```python
from build123d import *

# Parameters (mm, degrees)
BOSS_EXTRUDE1_DEPTH     = 5
BOSS_EXTRUDE2_DEPTH     = 2.5
CUT_EXTRUDE1_DEPTH      = 150.653904127
CUT_EXTRUDE1_DEPTH_BACK = 150.653904127


with BuildPart() as part:
    # Sketch1 → Boss-Extrude1 (new, symmetric)
    # profile 1 of 2: a face of its own
    with BuildSketch(Plane.XY):
        with BuildLine():
            Line((56.958357345, 16.35690948), (91.94062397, 26.262392372))
            ThreePointArc((91.94062397, 26.262392372), (58.546836742, 40.020208922), (27.617225647, 21.371302811))
            ThreePointArc((27.617225647, 21.371302811), (21.454195768, 0), (27.617225647, -21.371302811))
            ThreePointArc((27.617225647, -21.371302811), (58.546836742, -40.020208922), (91.94062397, -26.262392372))
            Line((91.94062397, -26.262392372), (107.630769277, -4.631577729))
            Line((107.630769277, -4.631577729), (66.221512803, -16.35690948))
            ThreePointArc((66.221512803, -16.35690948), (45.233025594, -4.631577729), (56.958357345, 16.35690948))
        make_face()
    # profile 2 of 2: a face of its own
    with BuildSketch(Plane.XY):
        with BuildLine():
            ThreePointArc((27.617225647, -21.371302811), (21.454195768, 0), (27.617225647, 21.371302811))
            ThreePointArc((27.617225647, 21.371302811), (20.358110781, 14.513813118), (10.688318885, 12.02081528))
            Line((10.688318885, 12.02081528), (-112.81430605, 12.02081528))
            ThreePointArc((-112.81430605, 12.02081528), (-114.76520927, 12.212962476), (-116.641140374, 12.782019955))
            Line((-116.641140374, 12.782019955), (-126.824245004, 17))
            Line((-126.824245004, 17), (-138.845060284, 12.02081528))
            Line((-138.845060284, 12.02081528), (-143.824245004, 0))
            Line((-143.824245004, 0), (-138.845060284, -12.02081528))
            Line((-138.845060284, -12.02081528), (-126.824245004, -17))
            Line((-126.824245004, -17), (-116.641140374, -12.782019955))
            ThreePointArc((-116.641140374, -12.782019955), (-114.76520927, -12.212962476), (-112.81430605, -12.02081528))
            Line((-112.81430605, -12.02081528), (10.688318885, -12.02081528))
            ThreePointArc((10.688318885, -12.02081528), (20.358110781, -14.513813118), (27.617225647, -21.371302811))
        make_face()
        with BuildLine():
            ThreePointArc((-61.622122108, -6.728166576), (-68.350288684, 0), (-61.622122108, 6.728166576))
            Line((-61.622122108, 6.728166576), (-32.694798011, 6.728166576))
            ThreePointArc((-32.694798011, 6.728166576), (-25.966631435, 0), (-32.694798011, -6.728166576))
            Line((-32.694798011, -6.728166576), (-61.622122108, -6.728166576))
        make_face(mode=Mode.SUBTRACT)
    extrude(amount=BOSS_EXTRUDE1_DEPTH, both=True)

    # Sketch1_3 → Boss-Extrude2 (add, symmetric)
    with BuildSketch(Plane.XY):
        with BuildLine():
            Line((-61.622122108, -6.728166576), (-32.694798011, -6.728166576))
            ThreePointArc((-32.694798011, -6.728166576), (-25.966631435, 0), (-32.694798011, 6.728166576))
            Line((-32.694798011, 6.728166576), (-61.622122108, 6.728166576))
            ThreePointArc((-61.622122108, 6.728166576), (-68.350288684, 0), (-61.622122108, -6.728166576))
        make_face()
    extrude(amount=BOSS_EXTRUDE2_DEPTH, both=True)

    # Sketch2 → Cut-Extrude1 (cut, two sides: drawn at the far end of the back side and taken through both)
    with BuildSketch(Plane.XY.offset(5).offset(-CUT_EXTRUDE1_DEPTH_BACK)):
        Polygon((-126.824245004, 13.306981608), (-136.233701936, 9.409456932), (-140.131226612, 0), (-136.233701936, -9.409456932), (-126.824245004, -13.306981608), (-117.414788072, -9.409456932), (-113.517263396, 0), (-117.414788072, 9.409456932), align=None)
    extrude(amount=CUT_EXTRUDE1_DEPTH + CUT_EXTRUDE1_DEPTH_BACK, mode=Mode.SUBTRACT)


solid = part.part
```
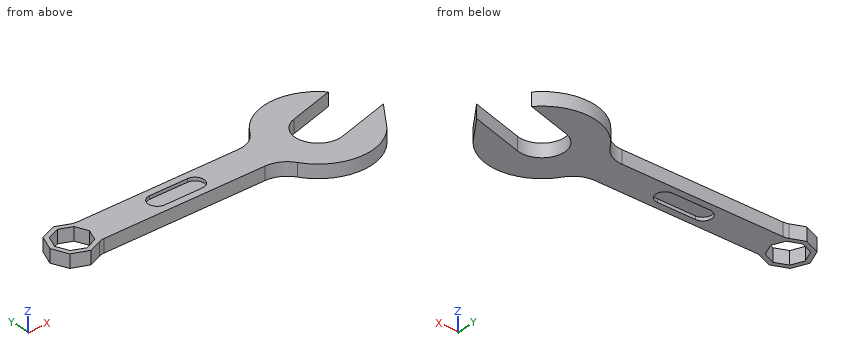
Work out the finished part from the listing and answer in its coordinate system (mm). Give positions to 0.01 mm unless a question says otherwise; leave off trailing zeros. Loops run counter-clockwise (first coordinate to the right, second up) from the corner with the lowest first, then second, coordinate; pieces in that order, holes last. Notation, with made-up numbers: (8.5, -14.75) - (34.5, -14.75) arc R17 ccw to (34.5, 18.25) - close; hole circle Ø3 at (89.25, 53). An arc over 180 degrees is marked (long way). Use CSV: the item, a comma, the result in double quotes. Start each with the question number.
(1) Find section D-D, the plane x = -104.5. Determine the outline of the cut face in (y, z).
(2) Find the intervals of material crossed by L1, parallel to Y at x = -62, z = 1.25; L2, parallel to Y at x = -127, z = 4.75; L3, parallel to X at y = 15, z = -2.25, in increasing order.
(3) Each of these flat-tipped pins is pushed along its axis until it touches: pin 1 (3 mm diameter, centred on x = -30.5, z = -1.5, fed in from +Y); pin 2 (6.5 mm diameter, centred on x = -41.5, y = -2.5, fed in from -Z); pin 3 (1.2 mm diameter, centred on x = -44.5, z = -4.5, fed in from -Y). Where does it stop, or does it pass through?
(4) Find section C-C, the plane x = -50.5. Determine the outline of the cut face in (y, z), plus the area to 3 significant figures.
(5) Find section A-A, the plane z = -0.75. Determine the outline of the cut face in (x, y), plus the area to 3 significant figures.
(6) Find section B-B, the plane y = -2.5. Determine the outline of the cut face in (x, z).
Results found:
1,outline,"(-12.02, -5) - (12.02, -5) - (12.02, 5) - (-12.02, 5) - close"
2,L1,"-12.02 to 12.02"
2,L2,"-16.93 to -13.23, 13.23 to 16.93"
2,L3,"-131.65 to -122, 21.19 to 53.59"
3,pin 1,"y = 12.02"
3,pin 2,"z = -2.5"
3,pin 3,"y = -12.02"
4,outline,"(-12.02, -5) - (-6.73, -5) - (-6.73, -2.5) - (6.73, -2.5) - (6.73, -5) - (12.02, -5) - (12.02, 5) - (6.73, 5) - (6.73, 2.5) - (-6.73, 2.5) - (-6.73, 5) - (-12.02, 5) - close"
4,area,"173 mm^2"
5,outline,"(-143.82, 0) - (-138.85, -12.02) - (-126.82, -17) - (-116.64, -12.78) arc R10 cw to (-112.81, -12.02) - (10.69, -12.02) arc R20 cw to (27.62, -21.37) arc R40.14 ccw to (91.94, -26.26) - (107.63, -4.63) - (66.22, -16.36) arc R17 cw to (56.96, 16.36) - (91.94, 26.26) arc R40.14 ccw to (27.62, 21.37) arc R20 cw to (10.69, 12.02) - (-112.81, 12.02) arc R10 cw to (-116.64, 12.78) - (-126.82, 17) - (-138.85, 12.02) - close; hole (-140.13, 0) - (-136.23, -9.41) - (-126.82, -13.31) - (-117.41, -9.41) - (-113.52, 0) - (-117.41, 9.41) - (-126.82, 13.31) - (-136.23, 9.41) - close"
5,area,"6,910 mm^2"
6,outline,"(-142.79, -5) - (-139.1, -5) - (-139.1, 5) - (-142.79, 5) - close; (-114.55, -5) - (-67.87, -5) - (-67.87, -2.5) - (-26.45, -2.5) - (-26.45, -5) - (44.77, -5) - (44.77, 5) - (-26.45, 5) - (-26.45, 2.5) - (-67.87, 2.5) - (-67.87, 5) - (-114.55, 5) - close"
